Autodesk Inventor part; units mm, degrees
ref_plane "YZ Plane" through (0, 0, 0) normal (1, 0, 0) x (0, 1, 0)
ref_plane "XZ Plane" through (0, 0, 0) normal (0, 1, 0) x (-1, 0, 0)
ref_plane "XY Plane" through (0, 0, 0) normal (0, 0, 1) x (1, 0, 0)
sketch "스케치1" plane through (0, 0, 0) normal (0, 0, 1) x (1, 0, 0)
  line L0 (0, 0) -> (19.3, 0)
  line L1 (19.3, 0) -> (19.3, 9)
  line L2 (19.3, 9) -> (10.3, 9)
  line L3 (0, 9) -> (0, 0)
  line L4 (10.3, 9) -> (10.3, 16.3)
  line L5 (10.3, 16.3) -> (0, 16.3)
  line L6 (0, 16.3) -> (0, 9)
  dimension "d0" = 9
  dimension "d1" = 19.3
  dimension "d2" = 16.3
  dimension "d3" = 10.3
extrude "돌출1" add sketch "스케치1" along normal blind 1.8
fillet "모깎기1" radius 2 1 edges at (10.3, 9, 0.9)
sketch "스케치2" plane through (0, 0, 1.8) normal (0, 0, 1) x (1, 0, 0)
  line L0 (18.5, 0.3) -> (4, 0.3)
  line L1 (4, 0.3) -> (4, 5.1)
  line L2 (4, 5.1) -> (18.5, 5.1)
  line L3 (18.5, 5.1) -> (18.5, 0.3)
  line L4 (19.3, 0) -> (19.3, 9)
  line L5 (0, 0) -> (19.3, 0)
  line L6 (4, 2.8) -> (4, 2.8)
  line L7 (6.5, 0.3) -> (6.5, 0.3)
  line L8 (6.5, 0.3) -> (16, 0.3)
  line L9 (16, 0.3) -> (16, 0.3)
  line L10 (18.5, 2.8) -> (18.5, 2.8)
  arc A0 (6.5, 0.3) -> (4, 2.8) centre (4, 0.3) ccw
  arc A1 (18.5, 2.8) -> (16, 0.3) centre (18.5, 0.3) ccw
  point P0 (6.5, 2.8)
  point P1 (16, 2.8)
  dimension "d7" = 0.8
  dimension "d8" = 14.5
  dimension "d9" = 4.8
  dimension "d10" = 0.3
  dimension "d11" = 2.3
  dimension "d12" = 2.5
  dimension "d13" = 2.5
  dimension "d14" = 2.5
  dimension "d15" = 2.5
extrude "돌출2" add sketch "스케치2" along normal blind 12.6 contours L0 A0 L1 L2 L3 A1
extrude "돌출3" add sketch "스케치2" along normal blind 1.8 contours L0 A1 L3 | L0 L1 A0
sketch "스케치3" plane through (0, 0, 1.8) normal (0, 0, 1) x (1, 0, 0)
  line L0 (1.15, 16.1) -> (9.15, 16.1)
  line L1 (9.15, 16.1) -> (9.15, 12.1)
  line L2 (9.15, 12.1) -> (1.15, 12.1)
  line L3 (1.15, 12.1) -> (1.15, 16.1)
  line L4 (10.3, 16.3) -> (0, 16.3)
  point P0 (0, 0)
  point P1 (5.15, 16.1)
  point P2 (5.15, 16.3)
  dimension "d20" = 8
  dimension "d21" = 4
  dimension "d22" = 0.2
extrude "돌출4" add sketch "스케치3" along normal blind 4.25
properties part number "HDMI_Port"
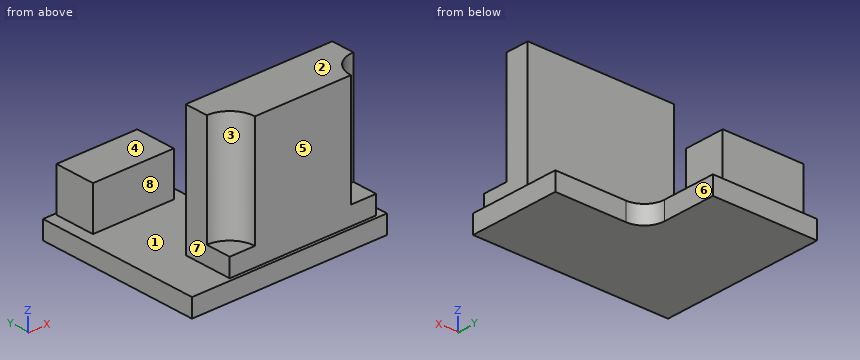
CAD build for the part. Positions are in the model's coordinates, mm. Face numbers are marked on the shaded views. A direction names the side the tool comes from. Round coordinates to 2 decimals unless told otherwise and drop trailing zeros. Order: outer loops, then holes, each group sorted by start corner. A loop starts at its lowest first (then second) coordinate and runs counter-clockwise, first axis right, second up. Notation, with made-up numbers: (50.5, 63.5) -> (89.5, 63.5) arc R8 cw to (89.5, 72.5) -> close; hole circle Ø11 at (36, 3.25). An arc over 180 degrees is marked (long way). Write item = value, one per line. Start each with the question number.
(1) Probe line 1 (Y direction, x = 15.75, z = 2.5); line 2 (Z direction, x = 3.25, y = 9.25); line 3 (Y direction, x = 2, z = 5). List the from-to ranges inside material, lowest first. Write a range as [from, to].
(2) Cut at C-C, the plane z = 5.5. List the corners of the cut face in (x, y).
(3) Pull direction Y, two halves, no side cores. Call the marked faces 1, 2 and 3: released by +Y, released by -Y, zero draft, split by the parting line, or undercut.
(4) Cut at B-B, the plane x = 8. List the corners of the cut face in (y, z), then the cut area to 3 significant figures.
(5) Cut at A-A, the plane z = 2.25. List the corners of the cut face in (x, y), then the cut area to 3 significant figures.
(6) Cut at D-D, the plane y = 12.5. List the corners of the cut face in (x, z), then the cut area to 3 significant figures.
(7) Pin check, flat tips, straight feed: P1, Ø4, axis at x = 13.5, z = 5.5, coming from the +Y side; P2, Ø1.4, axis at x = 15.5, z = 1, coming from the +Y side; P3, Ø2, axis at y = 14, z = 1, coming from the +X side. Stop position of each tip, or through.
(8) Which spindle directions (+Z, -Z, +X, -X, +Y, -Y) get a long thin tool onto all of the face, cutting with end or side? Do the marked faces 4, 5, 6, 7 and 8. Say none if no direction does.
Model answer:
q1.line_1 = [0.3, 5.1]
q1.line_2 = [0, 1.8]
q1.line_3 = [12.1, 16.1]
q2.outline = (1.15, 12.1) -> (9.15, 12.1) -> (9.15, 16.1) -> (1.15, 16.1) -> close; (4, 2.8) arc R2.5 cw to (6.5, 0.3) -> (16, 0.3) arc R2.5 cw to (18.5, 2.8) -> (18.5, 5.1) -> (4, 5.1) -> close
q3.face_1 = undercut
q3.face_2 = zero draft
q3.face_3 = released by -Y
q4.outline = (0, 0) -> (16.3, 0) -> (16.3, 1.8) -> (16.1, 1.8) -> (16.1, 6.05) -> (12.1, 6.05) -> (12.1, 1.8) -> (5.1, 1.8) -> (5.1, 14.4) -> (0.3, 14.4) -> (0.3, 1.8) -> (0, 1.8) -> close
q4.area = 107 mm2
q5.outline = (1.15, 12.1) -> (9.15, 12.1) -> (9.15, 16.1) -> (1.15, 16.1) -> close; (4, 0.3) -> (18.5, 0.3) -> (18.5, 5.1) -> (4, 5.1) -> close
q5.area = 102 mm2
q6.outline = (0, 0) -> (10.3, 0) -> (10.3, 1.8) -> (9.15, 1.8) -> (9.15, 6.05) -> (1.15, 6.05) -> (1.15, 1.8) -> (0, 1.8) -> close
q6.area = 52.5 mm2
q7.P1 = 5.1
q7.P2 = 9
q7.P3 = 10.3
q8.face_4 = +Z, +X, -X, +Y
q8.face_5 = +Z, +X, -X, -Y
q8.face_6 = +Z, -Z, +X, +Y
q8.face_7 = +Z, -X, -Y
q8.face_8 = +Z, +X, -X
